Geometry: final body of the model. Coordinates: model frame, mm. Round coordinates to 2 decimals unless told otherwise and drop trailing zeros. Order: outer loops, then holes, each group sorted by start corner. A loop starts at its lowest first (then second) coordinate and runs counter-clockwise, first axis right, second up. Notation, with made-up numbers: M 42,70.5 L 76,70.5 A29 ccw 76,98.5 Z; hole C 68.25,79 d3. An arc over 180 degrees is marked long. Put each result on its own line as item: value. Start each with the question number.
1) Draft query along Z for faces 1 (the cylindrical face through (7.509, 0.986, 23.846)), 2 (the cylindrical face through (-0.766, 1.014, -20.154)), 3 (the flat face through (0, 2, 0)). Return one class per face: pulls with the +Z half, pulls with the -Z half, needs draft (parallel to the pull), parting line crosses it, or undercut.
2) Section C-C, the plane y = 1.5. Return loops of the section in (x, z).
3) Material intervals for probe 1 along X at (y, z) = (1.35, 0); probe 2 along Z at (x, y) = (-1, 0.65); probe 3 along X at (y, z) = (1.35, 15), sorted ascending. Write a range as [from, to].
4) Section A-A, the plane x = 0. Return loops of the section in (y, z), then the cut area to 3 significant figures.
5) Section B-B, the plane z = 0. Return loops of the section in (x, y).
6) Section D-D, the plane x = -22. Return loops of the section in (y, z).
from build123d import *

# Parameters (mm, degrees)
IZIM1_R                     = 25
IZIM1_R_2                   = 2
Y_KSEKLIK_EKSTR_ZYON1_DEPTH = 2
IZIM3_R                     = 1.998800289
KES_EKSTR_ZYON1_DEPTH       = 2


with BuildPart() as part:
    # Çizim1 → Yükseklik-Ekstrüzyon1 (new body)
    with BuildSketch(Plane(origin=(0, 0, 0), x_dir=(1, 0, 0), z_dir=(0, 1, 0))):
        with Locations(Location((0, 0, 0), (0, 0, 270))):
            Circle(IZIM1_R)
        with Locations(Location((-22, 0, 0), (0, 0, 270))):
            Circle(IZIM1_R_2, mode=Mode.SUBTRACT)
        with Locations(Location((22, 0, 0), (0, 0, 270))):
            Circle(IZIM1_R_2, mode=Mode.SUBTRACT)
    extrude(amount=Y_KSEKLIK_EKSTR_ZYON1_DEPTH)

    # Çizim3 → Kes-Ekstrüzyon1 (cut)
    with BuildSketch(Plane(origin=(0, 2, 0), x_dir=(1, 0, 0), z_dir=(0, 1, 0))):
        with Locations(Location((0, 22, 0), (0, 0, 270))):
            Circle(IZIM3_R)
        with Locations(Location((0, -22, 0), (0, 0, 270))):
            Circle(IZIM3_R)
    extrude(amount=-KES_EKSTR_ZYON1_DEPTH, mode=Mode.SUBTRACT)


solid = part.part
Result sheet:
1. face 1: parting line crosses it
1. face 2: undercut
1. face 3: needs draft
2. outline: C 0,0 d50; hole C -22,0 d4; hole C 0,-22 d4; hole C 0,22 d4; hole C 22,0 d4
3. probe 1: x = [-25, -24], [-20, 20], [24, 25]
3. probe 2: z = [-24.98, -23.73], [-20.27, 20.27], [23.73, 24.98]
3. probe 3: x = [-20, 20]
4. outline: M 0,-25 L 2,-25 L 2,-24 L 0,-24 Z; M 0,-20 L 2,-20 L 2,20 L 0,20 Z; M 0,24 L 2,24 L 2,25 L 0,25 Z
4. area: 84.0 mm2
5. outline: M -25,0 L -24,0 L -24,2 L -25,2 Z; M -20,0 L 20,0 L 20,2 L -20,2 Z; M 24,0 L 25,0 L 25,2 L 24,2 Z
6. outline: M 0,-11.87 L 2,-11.87 L 2,-2 L 0,-2 Z; M 0,2 L 2,2 L 2,11.87 L 0,11.87 Z
